Could you check a few things on this drawing? It's one solid part, dimensions in mm from its lowest x, y, z. A direction names the side the tool comes from. Give positions to 0.01 mm unless a question says otherwise; leave off trailing zeros. Order: outer loops, then holes, each group sorted by start corner. A loop starts at its lowest first (then second) coordinate and runs counter-clockwise, first axis right, second up.
Item 1: Which directions (+Z, -Z, +X, -X, +Y, -Y) give clear straight access to the entire face, cutting with the end or side of a thin tool? Please do the marked faces 1, 2 and 3.
Item 2: If I drill on line 1 along Y through (x, z) = (8, 3); line 2 along Z through (x, y) = (12, 9.25) (1 decimal), over which ranges is the centre line in solid material (lowest first)?
Item 3: I'm going to push flat-ended pins straight in: pin 1 Ø5 at (y, z) = (8.5, 10.5) entering from +X; pin 2 Ø1.5 at (x, z) = (5.5, 5) entering from +Y; pin 3 Ø5 at (y, z) = (4.5, 13) entering from -X. Where does each tip first touch, or does it pass through?
Item 4: I want a section at D-D, the plane x = 1.25. Write out the boundary of the cut face in (y, z), then the cut area to 3 significant figures.
Item 5: I want a section at B-B, the plane z = 12. Write out the boundary of the cut face in (x, y), then the cut area to 3 significant figures.
Item 6: I want a section at A-A, the plane x = 7.5. Write out the boundary of the cut face in (y, z).
Item 7: I want a section at C-C, the plane y = 7.5. Write out the boundary of the cut face in (x, z), then the cut area to 3 significant figures.
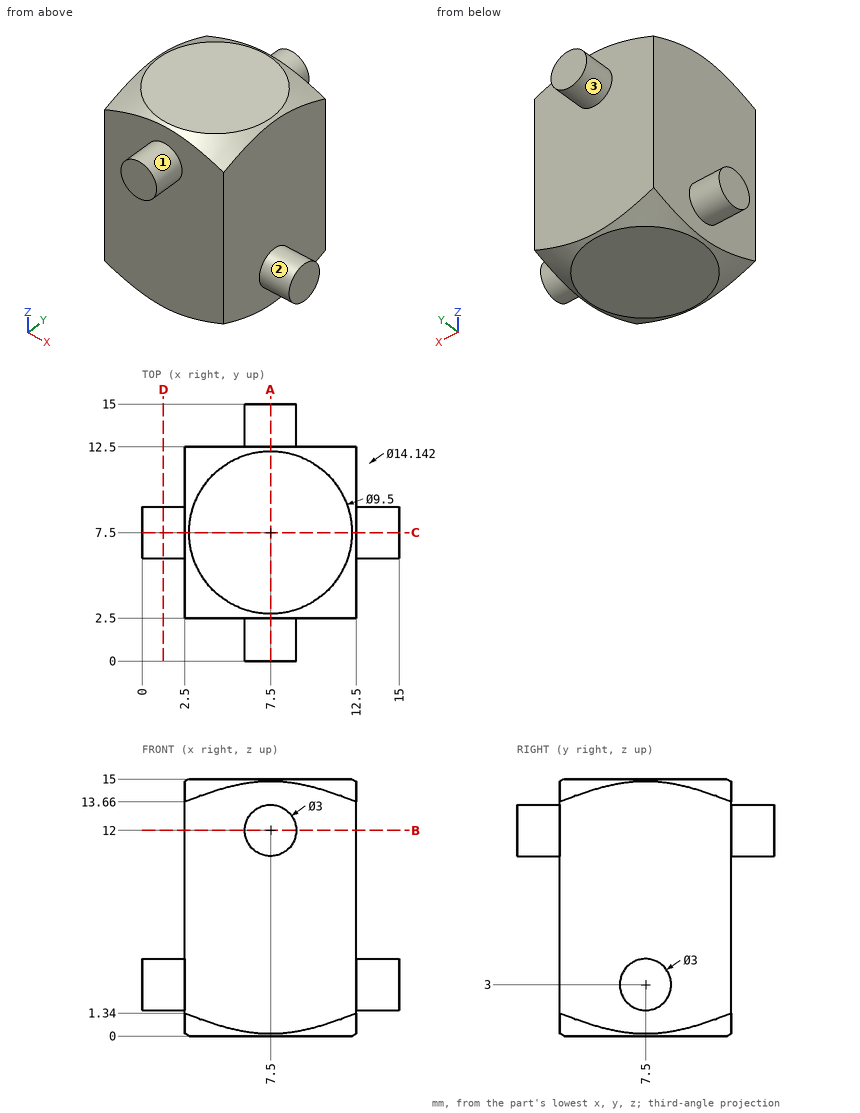
Results list:
1. face 1: -Y
1. face 2: +X
1. face 3: +Y
2. line 1: y = 2.5 to 12.5
2. line 2: z = 0 to 15
3. pin 1: stops at x = 12.5
3. pin 2: stops at y = 12.5
3. pin 3: stops at x = 2.5
4. outline: circle Ø3 at (7.5, 3)
4. area: 7.07 mm2
5. outline: (2.5, 2.5) - (6, 2.5) - (6, 0) - (9, 0) - (9, 2.5) - (12.5, 2.5) - (12.5, 12.5) - (9, 12.5) - (9, 15) - (6, 15) - (6, 12.5) - (2.5, 12.5) - close
5. area: 115 mm2
6. outline: (0, 10.5) - (2.5, 10.5) - (2.5, 0.14) - (2.75, 0) - (12.25, 0) - (12.5, 0.14) - (12.5, 10.5) - (15, 10.5) - (15, 13.5) - (12.5, 13.5) - (12.5, 14.86) - (12.25, 15) - (2.75, 15) - (2.5, 14.86) - (2.5, 13.5) - (0, 13.5) - close
7. outline: (0, 1.5) - (2.5, 1.5) - (2.5, 0.14) - (2.75, 0) - (12.25, 0) - (12.5, 0.14) - (12.5, 1.5) - (15, 1.5) - (15, 4.5) - (12.5, 4.5) - (12.5, 14.86) - (12.25, 15) - (2.75, 15) - (2.5, 14.86) - (2.5, 4.5) - (0, 4.5) - close
7. area: 165 mm2
